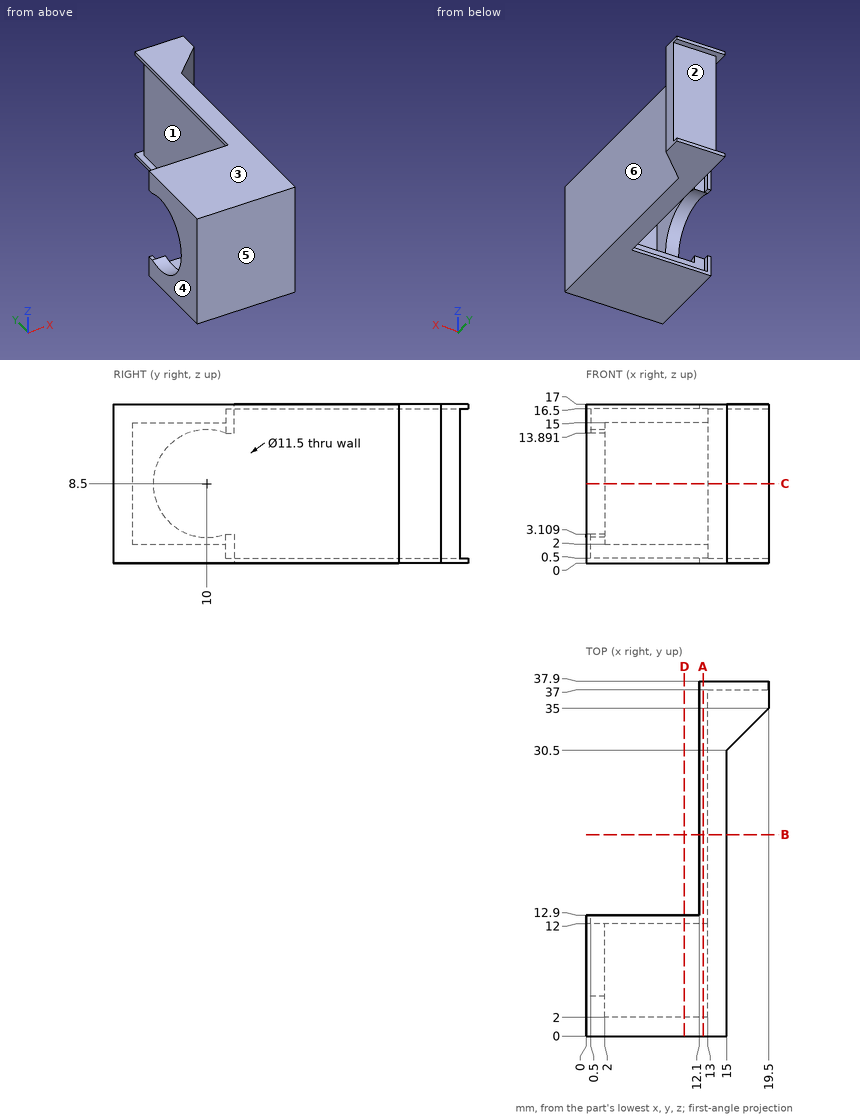
Here's the drawing with two shaded views (mm, measured from the low corner). I have some questions. A direction names the side the tool comes from. Give positions to 0.01 mm unless a question says otherwise; leave off trailing zeros. Loops run counter-clockwise (first coordinate to the right, second up) from the corner with the lowest first, then second, coordinate; pieces in that order, holes last. Notation, with made-up numbers: (17, 22) -> (36, 22) arc R13 cw to (36, 31) -> close; hole circle Ø6 at (-39.75, 70.5). An arc over 180 degrees is marked (long way). One line per item, written item: value.
Q1. Suppose I cut it at A-A on x = 12.5. Please give me the cut outline in (y, z), then the cut area to 3 significant figures.
Answers follow:
outline: (0, 0) -> (37.9, 0) -> (37.9, 0.5) -> (12, 0.5) -> (12, 2) -> (2, 2) -> (2, 15) -> (12, 15) -> (12, 16.5) -> (37.9, 16.5) -> (37.9, 17) -> (0, 17) -> close
area: 99.9 mm^2
Q2. We'd pull the mould along Z, two halves only. Please class the marked faces 1, 2, 3 and 4: pulls with the +Z half, pulls with the -Z half, needs draft (parallel to the pull), parting line crosses it, or undercut.
Answers follow:
face 1: undercut
face 2: undercut
face 3: pulls with the +Z half
face 4: needs draft
Q3. Suppose I cut it at C-C on z = 8.5. Please give me the cut outline in (x, y).
Answers follow:
outline: (0, 0) -> (15, 0) -> (15, 30.5) -> (19.5, 35) -> (19.5, 37) -> (13, 37) -> (13, 2) -> (2, 2) -> (2, 4.25) -> (0, 4.25) -> close
Q4. Suppose I cut it at B-B on y = 21.5. Please give me the cut outline in (x, z), then the cut area to 3 significant figures.
Answers follow:
outline: (12.1, 0) -> (15, 0) -> (15, 17) -> (12.1, 17) -> (12.1, 16.5) -> (13, 16.5) -> (13, 0.5) -> (12.1, 0.5) -> close
area: 34.9 mm^2
Q5. On a 3-axis mill with a long thin cutter (end or side, diameter ignored), from which of +Z, -Z, +X, -X, +Y, -Y can I reach the whole of each face in a straight line? I mean the marked faces 5 and 6. Say none if no direction works.
Answers follow:
face 5: +Z, -Z, +X, -X, -Y
face 6: +Z, -Z, +X, -Y
Q6. Suppose I cut it at D-D on x = 10.5. Please give me the cut outline in (y, z).
Answers follow:
outline: (0, 0) -> (12.9, 0) -> (12.9, 0.5) -> (12, 0.5) -> (12, 2) -> (2, 2) -> (2, 15) -> (12, 15) -> (12, 16.5) -> (12.9, 16.5) -> (12.9, 17) -> (0, 17) -> close
Q7. I'm going to push flat-ended pins straight in: pin 1 Ø5 at (x, z) = (15, 5.5) entering from +Y; pin 2 Ø2.5 at (x, z) = (3, 16) entering from +Y; pin 3 Ø1 at (y, z) = (26.5, 10) entering from +X. Where does each tip first touch, or does it pass through?
Answers follow:
pin 1: y = 37
pin 2: y = 12.9
pin 3: x = 15
Q8. If I drill on line 1 along X through (y, z) = (4.5, 6.5); line 2 along Z through (x, y) = (1.3, 10); line 3 along Z through (x, y) = (5.25, 3.5), over which ranges is the centre line in solid material (lowest first)?
Answers follow:
line 1: 0 to 2, 13 to 15
line 2: 0 to 2.75, 14.25 to 17
line 3: 0 to 2, 15 to 17
